```python
from build123d import *

# Parameters (mm, degrees)
BOSS_EXTRUDE1_DEPTH = 1.5748


with BuildPart() as part:
    # BPR2 PCB Outline → Boss-Extrude1 (new body)
    with BuildSketch(Plane.XY):
        with BuildLine():
            Line((83.596984325, 7.317563979), (83.596984325, 10.317563979))
            Line((83.596984325, 10.317563979), (103.596984325, 10.317563979))
            Line((103.596984325, 10.317563979), (103.596984325, 7.317563979))
            Line((103.596984325, 7.317563979), (121.040984325, 7.317563979))
            ThreePointArc((121.040984325, 7.317563979), (121.748091106, 7.610457198), (122.040984325, 8.317563979))
            Line((122.040984325, 8.317563979), (122.040984325, 66.317563979))
            ThreePointArc((122.040984325, 66.317563979), (121.748091106, 67.02467076), (121.040984325, 67.317563979))
            Line((121.040984325, 67.317563979), (56.570984325, 67.317563979))
            ThreePointArc((56.570984325, 67.317563979), (55.863877543, 67.02467076), (55.570984325, 66.317563979))
            Line((55.570984325, 66.317563979), (55.570984325, 7.317563979))
            Line((55.570984325, 7.317563979), (83.596984325, 7.317563979))
        make_face()
    extrude(amount=-BOSS_EXTRUDE1_DEPTH)


solid = part.part
```
The model under review builds one solid part; all positions refer to its coordinate system, in mm. A direction names the side the tool comes from. Round coordinates to 2 decimals unless told otherwise and drop trailing zeros. Write each loop counter-clockwise with the first axis right and the second up, starting at its lowest first coordinate (ties: lowest second). Pieces come first, ordered by that corner, then holes.
(1) Wall thickness on L1, parallel to Y at x = 87, z = -0.1: over which ranges is the line inside the solid? List them lowest first.
(2) We need section B-B on x = 97. Give the boundary of the cut face in (y, z), and give its area (3 significant figures).
(3) Mouldability with a two-part tool opening along X and no side actions: class faces 1 (the flat face through (55.571, 37, -1)), 2 (the flat face through (69, 7.318, -1)), 3 (the flat face through (103.597, 9, -1)) as +X half, -X half, draft (parallel to the pull), parting line (faces both ways), or undercut.
(4) Machinability: for faces 4 (the flat face through (93, 10.318, -1)), 5 (the flat face through (89, 67.318, -1)), which of the approach directions +Z, -Z, +X, -X, +Y, -Y give a long, thin tool a straight path to every point of the face, cutting with its end or side? Answer none if there is none.
(5) Insertion check: pin 1 (0.5 mm diameter, centred on x = 94.5, z = -1, fed in from -Y). The pin has a flat end and moves straight along its axis. Give the tip position at first contact, or say it passes through.
(6) We need section A-A on z = -1.2. Give the boundary of the cut face in (x, y), and give its area (3 significant figures).
Findings below:
1. L1: y = 10.32 to 67.32
2. outline: (10.32, -1.57) - (67.32, -1.57) - (67.32, 0) - (10.32, 0) - close
2. area: 89.8 mm2
3. face 1: -X half
3. face 2: draft
3. face 3: undercut
4. face 4: +Z, -Z, -Y
4. face 5: +Z, -Z, +X, -X, +Y
5. pin 1: stops at y = 10.32
6. outline: (55.57, 7.32) - (83.6, 7.32) - (83.6, 10.32) - (103.6, 10.32) - (103.6, 7.32) - (121.04, 7.32) arc R1 ccw to (122.04, 8.32) - (122.04, 66.32) arc R1 ccw to (121.04, 67.32) - (56.57, 67.32) arc R1 ccw to (55.57, 66.32) - close
6. area: 3,930 mm2
